Geometry: final body of the model. Coordinates: model frame, mm. Face numbers are marked on the shaded views. Give positions to 0.01 mm unless a question says otherwise; leave off trailing zeros. Write each loop counter-clockwise with the first axis right and the second up, starting at its lowest first coordinate (ties: lowest second). Pieces come first, ordered by that corner, then holes. Notation, with made-up numbers: M 32.5,62 L 79.5,62 A21 ccw 79.5,90 Z; hole C 22,28.25 d9. An arc over 180 degrees is marked long. Answer as a JSON object with one key per item and string values.
from build123d import *


with BuildPart() as part:
    # Schizzo1 → Rivoluzione1 (revolve)
    with BuildSketch(Plane.XY, mode=Mode.PRIVATE) as rivoluzione1_sk:
        with BuildLine():
            Line((-33, 0), (-36.5, 0))
            ThreePointArc((-36.5, 0), (-36.853553391, 0.146446609), (-37, 0.5))
            Line((-37, 0.5), (-37, 7.5))
            ThreePointArc((-37, 7.5), (-36.853553391, 7.853553391), (-36.5, 8))
            Line((-36.5, 8), (-33, 8))
            Line((-33, 8), (-30.814092893, 6.534380349))
            Line((-30.814092893, 6.534380349), (-30, 7.707960129))
            Line((-30, 7.707960129), (-30, 6.133062593))
            Line((-30, 6.133062593), (-30, 4.144217363))
            Line((-30, 4.144217363), (-33, 6.155674729))
            Line((-33, 6.155674729), (-33, 0))
        make_face()
    revolve(rivoluzione1_sk.sketch.rotate(Axis((0, 0, 0), (0, 1, 0)), 180), axis=Axis((0, 0, 0), (0, 1, 0)))


solid = part.part
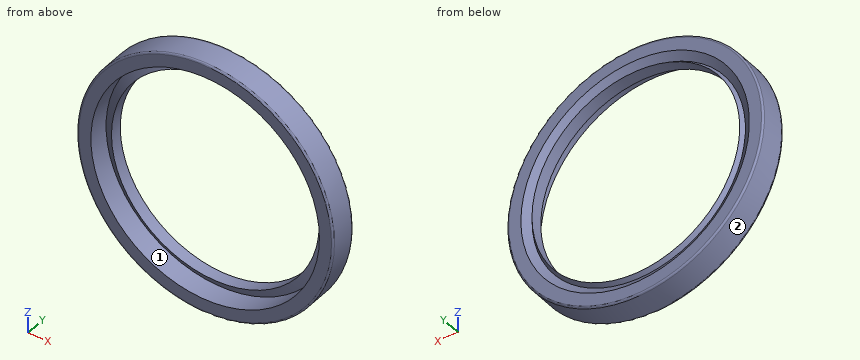
1) Contact query for flat-ended pins moving along their axis: P1, Ø2, axis at x = 29.5, y = 1, coming from the -Z side; P2, Ø2, axis at y = 6, z = -28.5, coming from the +X side. Output: stop coordinate, or through.
Geometry check:
{"P1": "stops at z = -23.6", "P2": "stops at x = 24.75"}
2) Line query: line 1 (Z direction, x = 0, y = 2.5); line 2 (Z direction, x = -20.5, y = 4.25); line 3 (Z direction, x = 0, y = 6.8). Output: solid intervals per line, ascending. Write a range as from..to.
Geometry check:
{"line 1": "z = -37..-33, 33..37", "line 2": "z = -30.8..-25.86, -22.12..-21.9, 21.9..22.12, 25.86..30.8", "line 3": "z = -37..-31.21, -30.63..-30, 30..30.63, 31.21..37"}
3) Pull-direction query (Z, two-part tool) for the marked faces 1 and 2; classes: pulls with the +Z half, pulls with the -Z half, needs draft (parallel to the pull), parting line crosses it, or undercut.
Geometry check:
{"face 1": "undercut", "face 2": "parting line crosses it"}
4) Cut plane A-A on z = 0. Return loops of the section in (x, y).
Geometry check:
{"outline": "M -37,0.5 A0.5 ccw -36.5,0 L -33,0 L -33,6.16 L -30,4.14 L -30,7.71 L -30.81,6.53 L -33,8 L -36.5,8 A0.5 ccw -37,7.5 Z; M 30,4.14 L 33,6.16 L 33,0 L 36.5,0 A0.5 ccw 37,0.5 L 37,7.5 A0.5 ccw 36.5,8 L 33,8 L 30.81,6.53 L 30,7.71 Z"}
5) Cut plane B-B on x = 0. Return loops of the section in (y, z).
Geometry check:
{"outline": "M 0,-36.5 A0.5 ccw 0.5,-37 L 7.5,-37 A0.5 ccw 8,-36.5 L 8,-33 L 6.53,-30.81 L 7.71,-30 L 4.14,-30 L 6.16,-33 L 0,-33 Z; M 0,33 L 6.16,33 L 4.14,30 L 7.71,30 L 6.53,30.81 L 8,33 L 8,36.5 A0.5 ccw 7.5,37 L 0.5,37 A0.5 ccw 0,36.5 Z"}
